Autodesk Fusion 360 part; units mm, degrees
sketch "Sketch1" plane through (0, 0, 0) normal (0, 0, 1) x (1, 0, 0)
  line L0 (0, 0) -> (-140, 0)
  line L1 (-140, 0) -> (-140, -160)
  line L2 (-140, -160) -> (0, -160)
  line L3 (0, -160) -> (0, 0)
  dimension "d1" = 140
  dimension "d2" = 160
extrude "Extrude1" add sketch "Sketch1" along normal blind 60
sketch "Sketch2" plane through (0, 0, 0) normal (0, 0, 1) x (1, 0, 0)
  line L0 (-140, 0) -> (-200, 0)
  line L1 (-200, 0) -> (-200, -100)
  line L2 (-200, -100) -> (-140, -100)
  line L3 (-140, -100) -> (-140, 0)
  dimension "d5" = 60
  dimension "d6" = 100
extrude "Extrude2" add sketch "Sketch2" along normal blind 60
sketch "Sketch3" plane through (0, 0, 0) normal (0, 0, 1) x (1, 0, 0)
sketch "Sketch4" plane through (0, 0, 0) normal (0, 0, 1) x (1, 0, 0)
  line L0 (-140, -160) -> (-200, -100)
  line L1 (-200, -100) -> (-140, -100)
  line L2 (-140, -100) -> (-140, -160)
extrude "Extrude3" add sketch "Sketch4" along normal blind 60
sketch "Sketch5" plane through (0, 0, 60) normal (0, 0, 1) x (-1, 0, 0)
  line L0 (0, 160) -> (0, 0)
  line L1 (0, 0) -> (200, 0)
  line L2 (200, 0) -> (200, 100)
  line L3 (200, 100) -> (140, 160)
  line L4 (140, 160) -> (0, 160)
  line L5 (0, 0) -> (20, 0)
  line L6 (20, 0) -> (20, 160)
  line L7 (20, 160) -> (0, 160)
  line L8 (0, 160) -> (0, 0)
  dimension "d11" = 20
extrude "Extrude4" add sketch "Sketch5" along normal blind 60 contours L0 L1 L4 L5 L6 L7 L8
sketch "Sketch6" plane through (0, 0, 60) normal (0, 0, 1) x (-1, 0, 0)
  line L0 (20, 160) -> (20, 0)
  line L1 (20, 0) -> (200, 0)
  line L2 (200, 0) -> (200, 100)
  line L3 (200, 100) -> (140, 160)
  line L4 (140, 160) -> (20, 160)
  line L5 (20, 0) -> (40, 0)
  line L6 (40, 0) -> (40, 140)
  line L7 (40, 140) -> (20, 140)
  line L8 (20, 140) -> (20, 0)
  dimension "d14" = 20
  dimension "d15" = 140
extrude "Extrude5" add sketch "Sketch6" along normal blind 60 contours L0 L1 L5 L6 L7 L8
sketch "Sketch7" plane through (0, 0, 60) normal (0, 0, 1) x (-1, 0, 0)
  line L0 (20, 140) -> (40, 140)
  line L1 (40, 140) -> (40, 0)
  line L2 (40, 0) -> (200, 0)
  line L3 (200, 0) -> (200, 100)
  line L4 (200, 100) -> (140, 160)
  line L5 (140, 160) -> (20, 160)
  line L6 (20, 160) -> (20, 140)
  line L7 (40, 140) -> (20, 160)
  line L8 (20, 140) -> (40, 140)
extrude "Extrude6" add sketch "Sketch7" along normal blind 60 contours L0 L6 L7 L8
sketch "Sketch8" plane through (0, 0, 60) normal (0, 0, 1) x (-1, 0, 0)
  line L0 (20, 160) -> (40, 140)
  line L1 (40, 140) -> (40, 0)
  line L2 (40, 0) -> (200, 0)
  line L3 (200, 0) -> (200, 100)
  line L4 (200, 100) -> (140, 160)
  line L5 (140, 160) -> (20, 160)
  line L6 (40, 0) -> (100, 0)
  line L7 (100, 0) -> (100, 80)
  line L8 (100, 80) -> (40, 80)
  line L9 (40, 80) -> (40, 0)
  dimension "d20" = 60
  dimension "d21" = 80
extrude "Extrude7" add sketch "Sketch8" along normal blind 40 contours L1 L2 L6 L7 L8 L9
sketch "Sketch9" plane through (0, 0, 60) normal (0, 0, 1) x (-1, 0, 0)
  line L0 (100, 80) -> (100, 0)
  line L1 (100, 0) -> (200, 0)
  line L2 (200, 0) -> (200, 100)
  line L3 (200, 100) -> (140, 160)
  line L4 (140, 160) -> (20, 160)
  line L5 (20, 160) -> (40, 140)
  line L6 (40, 140) -> (40, 80)
  line L7 (40, 80) -> (100, 80)
  line L8 (200, 0) -> (160, 0)
  line L9 (160, 0) -> (160, 20)
  line L10 (160, 20) -> (200, 20)
  line L11 (200, 20) -> (200, 0)
  dimension "d24" = 40
  dimension "d25" = 20
extrude "Extrude8" add sketch "Sketch9" along normal blind 40 contours L1 L2 L8 L9 L10 L11
sketch "Sketch10" plane through (0, 0, 60) normal (0, 0, 1) x (-1, 0, 0)
  line L0 (160, 0) -> (160, 20)
  line L1 (160, 20) -> (200, 20)
  line L2 (200, 20) -> (200, 100)
  line L3 (200, 100) -> (140, 160)
  line L4 (140, 160) -> (20, 160)
  line L5 (20, 160) -> (40, 140)
  line L6 (40, 140) -> (40, 80)
  line L7 (40, 80) -> (100, 80)
  line L8 (100, 80) -> (100, 0)
  line L9 (100, 0) -> (160, 0)
  line L10 (160, 20) -> (160, 0)
  line L11 (100, 0) -> (100, 80)
  line L12 (160, 20) -> (100, 80)
extrude "Extrude9" add sketch "Sketch10" along normal blind 40 contours L0 L8 L9 L10 L11 L12
sketch "Sketch11" plane through (-40, 0, 0) normal (-1, 0, 0) x (0, -1, 0)
  line L0 (0, 100) -> (80, 100)
  line L1 (80, 100) -> (80, 60)
  line L2 (80, 60) -> (140, 60)
  line L3 (140, 60) -> (140, 120)
  line L4 (140, 120) -> (0, 120)
  line L5 (0, 120) -> (0, 100)
sketch "Sketch12" plane through (-40, -70, 90) normal (-1, 0, 0) x (0, -1, 0)
  circle A0 centre (40, 0) radius 10
  dimension "d31" = 20
sketch "Sketch13" plane through (0, 0, 100) normal (0, 0, 1) x (-1, 0, 0)
  line L0 (40, 80) -> (40, 0)
  line L1 (40, 0) -> (200, 0)
  line L2 (200, 0) -> (200, 20)
  line L3 (200, 20) -> (160, 20)
  line L4 (160, 20) -> (100, 80)
  line L5 (100, 80) -> (40, 80)
  circle A0 centre (70, 40) radius 10
  dimension "d34" = 20
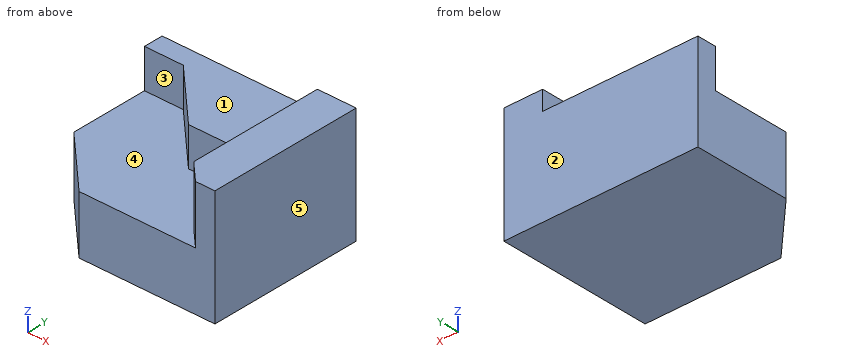
Geometry: final body of the model. Coordinates: model frame, mm. Face numbers are marked on the shaded views. A direction names the side the tool comes from. Coordinates: 2 decimals unless noted, no trailing zeros. Order: outer loops, then holes, each group sorted by start corner. A loop starts at its lowest first (then second) coordinate and runs counter-clockwise, first axis right, second up. Notation, with made-up numbers: M 63,82 L 107,82 A26 ccw 107,115 Z; hole C 28.5,-10.5 d7. An arc over 180 degrees is marked long. Answer in a Markdown table with one row per item. Add a question column.
Q1. Reachability of the marked faces 4 and 5 from +Z, -Z, +X, -X, +Y, -Y: full face, straight path, thin tool, end or side. Return the list, or none.
Q2. Section query A-A on y = -32. Return the cut outline in (x, z), and give its area (3 significant figures).
Q3. Mould query, pull axis Y, two halves, no side actions, for the marked faces 1, 2 and 3. Classes: released by +Y, released by -Y, zero draft, split by the parting line, or undercut.
Q4. Section query B-B on x = -121.5. Return the cut outline in (y, z).
Q5. Line query: L1, parallel to Y at x = -82, z = 62.5; L2, parallel to Y at x = -176.5, z = 96; L3, parallel to Z at x = -159, y = -42. Output: solid intervals per line, ascending.
Q6. Contact query for flat-ended pins moving along their axis: P1, Ø8, axis at x = -83.5, y = -24, coming from the +Z side; P2, Ø5, axis at y = -52.5, z = 95.5, coming from the -X side; P3, Ø8, axis at x = -173, z = 75.5, coming from the -Y side. Output: stop coordinate, or through.
Q7. Section query D-D on y = -55.5. Return the cut outline in (x, z), and give its area (3 significant figures).
Q8. Section query C-C on z = 56. Return the cut outline in (x, y), and give its area (3 significant figures).
Completed:
| question | item | result |
|---|---|---|
| 1 | face 4 | +Z, -X, -Y |
| 1 | face 5 | +Z, -Z, +X, +Y, -Y |
| 2 | outline | M -200,0 L 0,0 L 0,120 L -40,120 L -40,100 L -148,100 L -148,60 L -200,60 Z |
| 2 | area | 18,700 mm2 |
| 3 | face 1 | zero draft |
| 3 | face 2 | released by +Y |
| 3 | face 3 | released by -Y |
| 4 | outline | M -160,0 L 0,0 L 0,100 L -58.5,100 L -58.5,60 L -160,60 Z |
| 5 | L1 | y = -80 to 0 |
| 5 | L2 | y = -20 to 0 |
| 5 | L3 | z = 0 to 60 |
| 6 | P1 | stops at z = 100 |
| 6 | P2 | stops at x = -130 |
| 6 | P3 | stops at y = -20 |
| 7 | outline | M -200,0 L 0,0 L 0,120 L -40,120 L -40,100 L -124.5,100 L -124.5,60 L -200,60 Z |
| 7 | area | 17,800 mm2 |
| 8 | outline | M -200,-100 L -140,-160 L 0,-160 L 0,0 L -200,0 Z |
| 8 | area | 30,200 mm2 |
